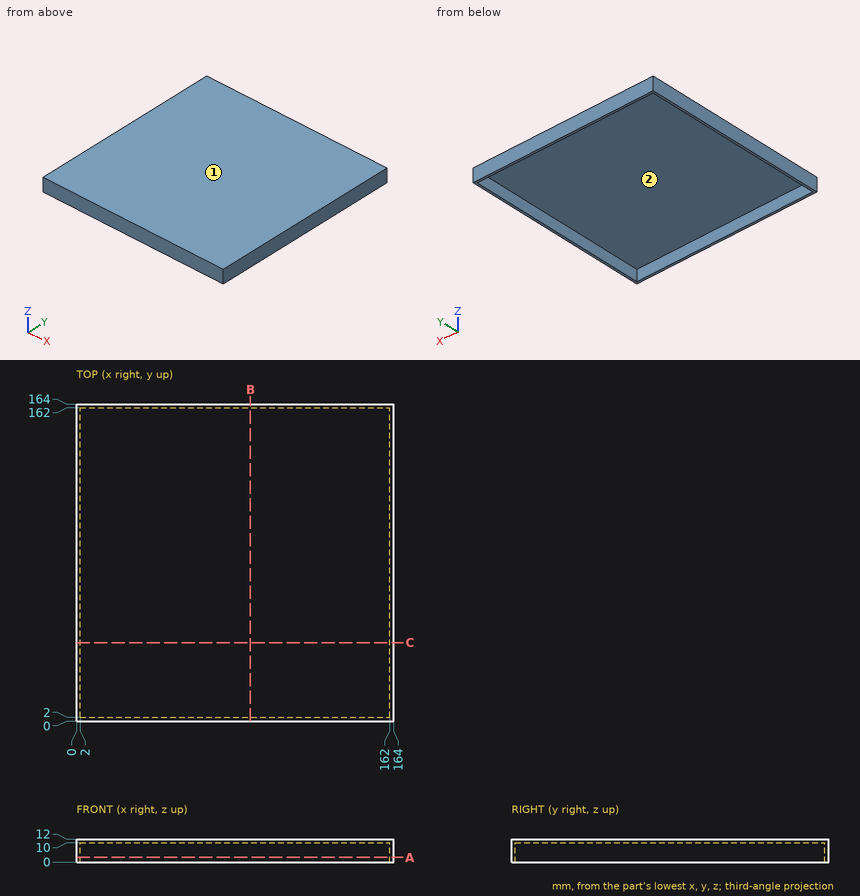
Source: three-view drawing plus pictorial views. Frame: mm from the lowest corner of the part. Round coordinates to 2 decimals unless told otherwise and drop trailing zeros. Write each loop counter-clockwise with the first axis right and the second up, starting at its lowest first coordinate (ties: lowest second). Pieces come first, ordered by that corner, then holes. Notation, with made-up numbers: M 70,47 L 107,47 A24 ccw 107,57 Z; hole C 66,76 d6. An arc over 180 degrees is marked long. One line per item, written item: value. Start each with the question number.
Item 1: Mould query, pull axis X, two halves, no side actions, for the marked faces 1 and 2. Classes: pulls with the +X half, pulls with the -X half, needs draft (parallel to the pull), parting line crosses it, or undercut.
Item 2: Section query B-B (x = 90). Return the cut outline in (y, z), plus the area to 3 significant figures.
Item 3: Pin query (flat end, axial travel): pin 1 (6 mm diameter, centred on x = 81, y = 73.5, fed in from -Z). Return the tip coordinate at first contact, or that it passes through.
Item 4: Section query A-A (z = 2.5). Return the cut outline in (x, y).
Item 5: Ray query, L1, parallel to X at y = 75, z = 9.5; L2, parallel to Z at x = 27.5, y = 38. Return the intervals inside material, ascending. Write a range as from..to.
Result set:
1. face 1: needs draft
1. face 2: undercut
2. outline: M 0,0 L 2,0 L 2,10 L 162,10 L 162,0 L 164,0 L 164,12 L 0,12 Z
2. area: 368 mm²
3. pin 1: stops at z = 10
4. outline: M 0,0 L 164,0 L 164,164 L 0,164 Z; hole M 2,2 L 162,2 L 162,162 L 2,162 Z
5. L1: x = 0..2, 162..164
5. L2: z = 10..12
